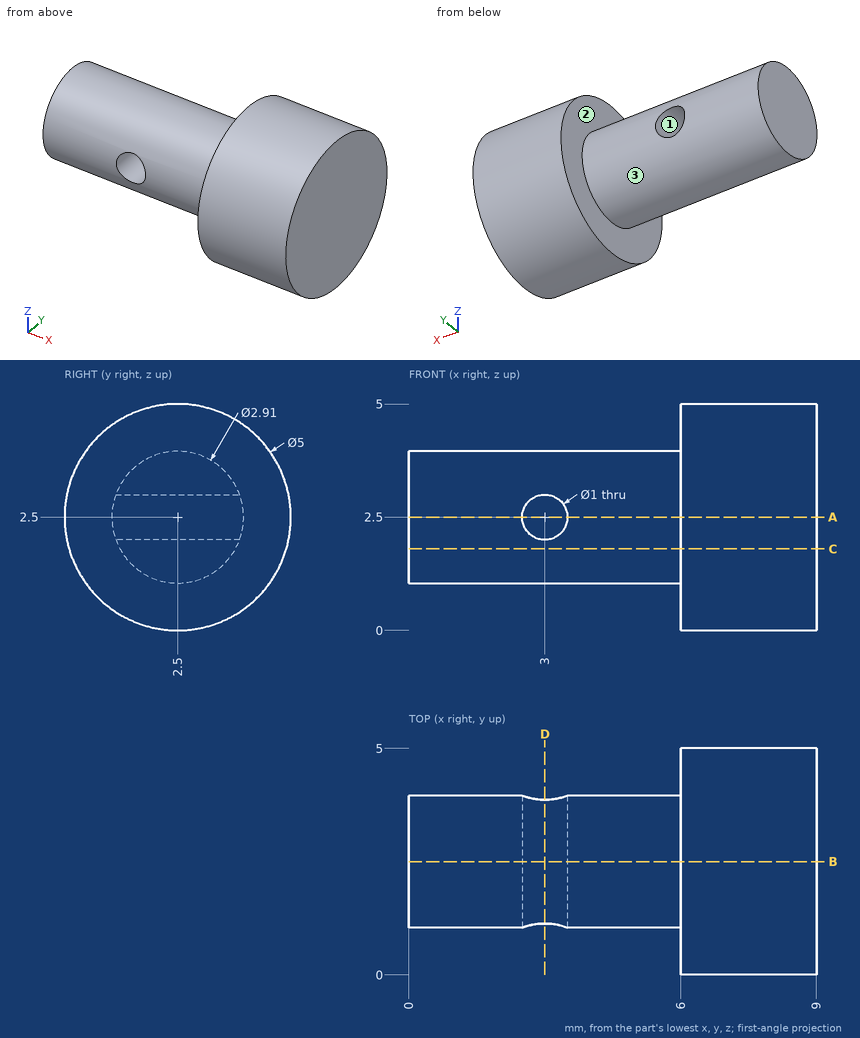
Study the drawing (mm; zero at the part's minimum x, y, z) and answer. Round coordinates to 2 decimals unless told otherwise and drop trailing zeros. Write each loop counter-clockwise with the first axis right and the second up, starting at its lowest first coordinate (ties: lowest second). Pieces come first, ordered by that corner, then holes. Notation, with made-up numbers: (75.25, -5.5) -> (104.25, -5.5) arc R33 cw to (104.25, 24.5) -> close; hole circle Ø6 at (-3, 78). An arc over 180 degrees is marked (long way). Write each question's results on one line, items separated by ' | '.
Item 1: A cutting plane is placed at C-C, the plane z = 1.8. Determine the outline of the cut face in (x, y).
Result set:
outline: (0, 1.22) -> (6, 1.22) -> (6, 0.1) -> (9, 0.1) -> (9, 4.9) -> (6, 4.9) -> (6, 3.78) -> (0, 3.78) -> close
Item 2: A cutting plane is placed at B-B, the plane y = 2.5. Determine the outline of the cut face in (x, z) (3 decimals).
Result set:
outline: (0, 1.045) -> (6, 1.045) -> (6, 0) -> (9, 0) -> (9, 5) -> (6, 5) -> (6, 3.955) -> (0, 3.955) -> close; hole circle Ø1 at (3, 2.5)
Item 3: Find the intervals of material crossed by line 1 along X through (y, z) = (2.7, 2.5); line 2 along X through (y, z) = (1.8, 0.85); line 3 along Z through (x, y) = (6.25, 2.4), in increasing order. Write a range as [from, to].
Result set:
line 1: [0, 2.5], [3.5, 9] | line 2: [6, 9] | line 3: [0, 5]
Item 4: A cutting plane is placed at D-D, the plane x = 3. Determine the outline of the cut face in (y, z) (3 decimals), plus the area to 3 significant figures.
Result set:
outline: (1.134, 2) arc R1.455 ccw to (3.866, 2) -> close; (1.134, 3) -> (3.866, 3) arc R1.455 ccw to start | area: 3.80 mm^2
Item 5: A cutting plane is placed at A-A, the plane z = 2.5. Determine the outline of the cut face in (x, y) (3 decimals).
Result set:
outline: (0, 1.045) -> (2.5, 1.045) -> (2.5, 3.955) -> (0, 3.955) -> close; (3.5, 1.045) -> (6, 1.045) -> (6, 0) -> (9, 0) -> (9, 5) -> (6, 5) -> (6, 3.955) -> (3.5, 3.955) -> close
Item 6: Flat-ended cylindrical pins translate along their axes: P1, Ø1, axis at x = 6.5, y = 4.5, coming from the -Z side; P2, Ø1.5, axis at x = 2, y = 1, coming from the +Z side; P3, Ø2, axis at x = 6.5, z = 4, coming from the -Y side. Find the tip coordinate at first contact, or state that the pin passes through.
Result set:
P1: z = 0.5 | P2: z = 3.75 | P3: y = 0.05
Item 7: The mould has two halves that part along Z. Classify the marked faces 1, 2 and 3: +Z half, -Z half, draft (parallel to the pull), parting line (faces both ways), or undercut.
Result set:
face 1: undercut | face 2: draft | face 3: parting line
